Can you work these out from the model? Positions are in its coordinate system, mm. Face numbers are marked on the shaded views. A direction names the side the tool comes from. Coordinates: 2 decimals unless noted, no trailing zeros. Loops run counter-clockwise (first coordinate to the right, second up) from the corner with the lowest first, then second, coordinate; pieces in that order, holes last.
```python
from build123d import *

# Parameters (mm, degrees)
F1_DEPTH = 25


with BuildPart() as f1:
    # F0 (on Front) → F1 (new body)
    with BuildSketch(Plane.XZ):
        with BuildLine():
            ThreePointArc((-89.145688, 80.140374), (-96.216756, 77.211442), (-99.145688, 70.140374))
            Line((-99.145688, 70.140374), (-99.145688, -69.859626))
            ThreePointArc((-99.145688, -69.859626), (-96.216756, -76.930694), (-89.145688, -79.859626))
            Line((-89.145688, -79.859626), (10.854312, -79.859626))
            ThreePointArc((10.854312, -79.859626), (17.92538, -76.930694), (20.854312, -69.859626))
            Line((20.854312, -69.859626), (20.854312, -59.859626))
            ThreePointArc((20.854312, -59.859626), (23.783244, -52.788558), (30.854312, -49.859626))
            Line((30.854312, -49.859626), (210.854312, -49.859626))
            ThreePointArc((210.854312, -49.859626), (217.92538, -46.930694), (220.854312, -39.859626))
            Line((220.854312, -39.859626), (220.854312, 40.140374))
            ThreePointArc((220.854312, 40.140374), (217.92538, 47.211442), (210.854312, 50.140374))
            Line((210.854312, 50.140374), (30.854312, 50.140374))
            ThreePointArc((30.854312, 50.140374), (23.783244, 53.069306), (20.854312, 60.140374))
            Line((20.854312, 60.140374), (20.854312, 70.140374))
            ThreePointArc((20.854312, 70.140374), (17.92538, 77.211442), (10.854312, 80.140374))
            Line((10.854312, 80.140374), (-89.145688, 80.140374))
        make_face()
        with BuildLine():
            ThreePointArc((-79.145688, -29.859626), (-76.216756, -22.788558), (-69.145688, -19.859626))
            Line((-69.145688, -19.859626), (-9.145688, -19.859626))
            ThreePointArc((-9.145688, -19.859626), (-2.07462, -22.788558), (0.854312, -29.859626))
            Line((0.854312, -29.859626), (0.854312, -49.859626))
            ThreePointArc((0.854312, -49.859626), (-2.07462, -56.930694), (-9.145688, -59.859626))
            Line((-9.145688, -59.859626), (-69.145688, -59.859626))
            ThreePointArc((-69.145688, -59.859626), (-76.216756, -56.930694), (-79.145688, -49.859626))
            Line((-79.145688, -49.859626), (-79.145688, -29.859626))
        make_face(mode=Mode.SUBTRACT)
        with BuildLine():
            ThreePointArc((19.293068, -29.859626), (22.222, -22.788558), (29.293068, -19.859626))
            Line((29.293068, -19.859626), (199.125637, -19.859626))
            ThreePointArc((199.125637, -19.859626), (206.196705, -22.788558), (209.125637, -29.859626))
            ThreePointArc((209.125637, -29.859626), (206.196705, -36.930694), (199.125637, -39.859626))
            Line((199.125637, -39.859626), (29.293068, -39.859626))
            ThreePointArc((29.293068, -39.859626), (22.222, -36.930694), (19.293068, -29.859626))
        make_face(mode=Mode.SUBTRACT)
        with BuildLine():
            ThreePointArc((-79.145688, 50.140374), (-76.216756, 57.211442), (-69.145688, 60.140374))
            Line((-69.145688, 60.140374), (-9.145688, 60.140374))
            ThreePointArc((-9.145688, 60.140374), (-2.07462, 57.211442), (0.854312, 50.140374))
            Line((0.854312, 50.140374), (0.854312, 30.140374))
            ThreePointArc((0.854312, 30.140374), (-2.07462, 23.069306), (-9.145688, 20.140374))
            Line((-9.145688, 20.140374), (-69.145688, 20.140374))
            ThreePointArc((-69.145688, 20.140374), (-76.216756, 23.069306), (-79.145688, 30.140374))
            Line((-79.145688, 30.140374), (-79.145688, 50.140374))
        make_face(mode=Mode.SUBTRACT)
        with BuildLine():
            ThreePointArc((18.76592, 0.140374), (21.694852, 7.211442), (28.76592, 10.140374))
            Line((28.76592, 10.140374), (199.125638, 10.140374))
            ThreePointArc((199.125638, 10.140374), (206.196706, 7.211442), (209.125638, 0.140373))
            ThreePointArc((209.125638, 0.140373), (206.196706, -6.930694), (199.125638, -9.859626))
            Line((199.125638, -9.859626), (28.76592, -9.859626))
            ThreePointArc((28.76592, -9.859626), (21.694852, -6.930694), (18.76592, 0.140374))
        make_face(mode=Mode.SUBTRACT)
        with BuildLine():
            Line((23.958503, 40.140374), (199.125637, 40.140374))
            ThreePointArc((199.125637, 40.140374), (205.417556, 37.912874), (208.906425, 32.222725))
            ThreePointArc((208.906425, 32.222725), (209.070683, 31.187303), (209.125637, 30.140374))
            ThreePointArc((209.125637, 30.140374), (209.061539, 29.00995), (208.870066, 27.894018))
            ThreePointArc((208.870066, 27.894018), (205.352051, 22.3153), (199.125637, 20.140374))
            Line((199.125637, 20.140374), (23.958503, 20.140374))
            ThreePointArc((23.958503, 20.140374), (16.887436, 23.069306), (13.958503, 30.140374))
            ThreePointArc((13.958503, 30.140374), (16.887436, 37.211442), (23.958503, 40.140374))
        make_face(mode=Mode.SUBTRACT)
    extrude(amount=F1_DEPTH)


solid = f1.part
```
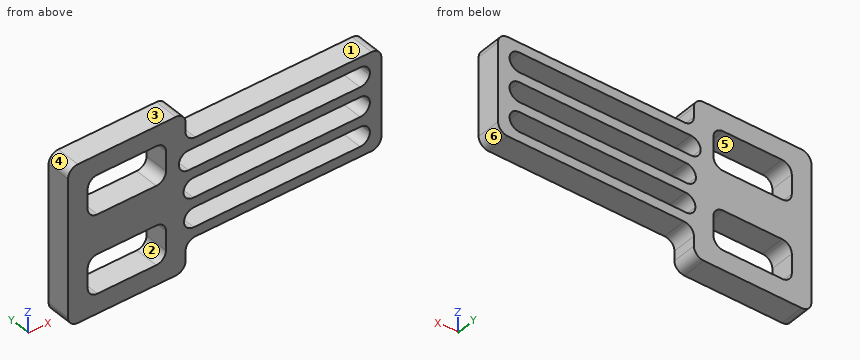
(1) I want a section at D-D on y = -20.5. State how many separate pieces and enclosed holes the cut face has, then the cut area to 3 significant figures.
Check values:
separate pieces: 1
enclosed holes: 5
area: 21,600 mm2
(2) I want a section at C-C on z = -56. Write out the boundary of the cut face in (x, y), then the cut area to 3 significant figures.
Check values:
outline: (-99.15, -25) - (-77.04, -25) - (-77.04, 0) - (-99.15, 0) - close; (-1.25, -25) - (21.63, -25) - (21.63, 0) - (-1.25, 0) - close
area: 1,120 mm2
(3) I want a section at A-A on x = -41. Write out the boundary of the cut face in (y, z).
Check values:
outline: (-25, -79.86) - (0, -79.86) - (0, -59.86) - (-25, -59.86) - close; (-25, -19.86) - (0, -19.86) - (0, 20.14) - (-25, 20.14) - close; (-25, 60.14) - (0, 60.14) - (0, 80.14) - (-25, 80.14) - close
(4) If we mould it in two halves opening along Z, with no side actions, what happens to the marked faces 4, 5 and 6? For each: released by +Z, released by -Z, zero draft, split by the parting line, or undercut.
Check values:
face 4: released by +Z
face 5: undercut
face 6: released by -Z
(5) I'm going to push flat-ended pins straight in: pin 1 (6 mm diameter, centred on x = 99.5, y = -4, fed in from +Z); pin 2 (10 mm diameter, centred on y = -12, z = -41.5, fed in from +X); pin 3 (1 mm diameter, centred on x = 131.5, y = -16, fed in from -Z); pin 4 (1 mm diameter, centred on y = -13.5, z = 60.5, fed in from +X). Where does each tip first touch, or does it pass through?
Check values:
pin 1: stops at z = 50.14
pin 2: stops at x = 220.85
pin 3: stops at z = -49.86
pin 4: stops at x = 20.86
(6) I want a section at B-B on x = 90. Write out the boundary of the cut face in (y, z), then the cut area to 3 significant figures.
Check values:
outline: (-25, -49.86) - (0, -49.86) - (0, -39.86) - (-25, -39.86) - close; (-25, -19.86) - (0, -19.86) - (0, -9.86) - (-25, -9.86) - close; (-25, 10.14) - (0, 10.14) - (0, 20.14) - (-25, 20.14) - close; (-25, 40.14) - (0, 40.14) - (0, 50.14) - (-25, 50.14) - close
area: 1,000 mm2
(7) If I drill on probe 1 along Z at (x, y) = (93, -17.25); probe 2 along Z at (x, y) = (-52, -6.75); probe 3 along X at (y, z) = (-9.75, -35.5), over which ranges is the centre line in solid material (lowest first)?
Check values:
probe 1: z = -49.86 to -39.86, -19.86 to -9.86, 10.14 to 20.14, 40.14 to 50.14
probe 2: z = -79.86 to -59.86, -19.86 to 20.14, 60.14 to 80.14
probe 3: x = -99.15 to -79.15, 0.85 to 21.04, 207.38 to 220.85
(8) Which directions (+Z, -Z, +X, -X, +Y, -Y) give clear straight access to the entire face, cutting with the end or side of a thin tool? Please do the marked faces 1, 2 and 3.
Check values:
face 1: +Z, +X, +Y, -Y
face 2: +Y, -Y
face 3: +Z, +X, -X, +Y, -Y
